Geometry: final body of the model. Coordinates: model frame, mm. Face numbers are marked on the shaded views. A direction names the side the tool comes from. Give positions to 0.01 mm unless a question says otherwise; leave off trailing zeros. Order: outer loops, then holes, each group sorted by start corner. A loop starts at its lowest first (then second) coordinate and runs counter-clockwise, first axis right, second up. Notation, with made-up numbers: (28.5, 45) -> (52.5, 45) arc R6 cw to (52.5, 50) -> close; hole circle Ø1 at (-7, 35.25). An arc over 180 degrees is marked (long way). One line per item, written item: value. Start each with the question number.
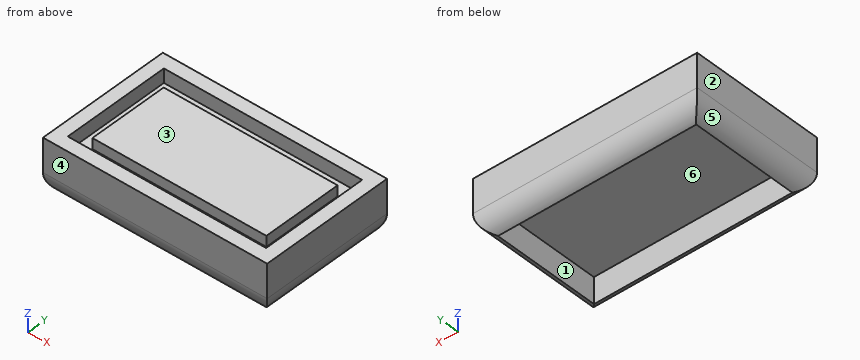
```python
from build123d import *

# Parameters (mm, degrees)
F0_W        = 50.8
F0_H        = 30.48
F0_W_2      = 44.9317246675
F0_H_2      = 24.4365520775
F1_DEPTH    = 6.35
F0_W_3      = 39.4137948751
F0_H_3      = 18.13034527
F2_DEPTH    = 3.175
F3_DEPTH    = 5.588
F4_T1_DEPTH = 76.2
F4_T3_DEPTH = 55.88


# Not quite as in the source:
# - a fillet or chamfer that OpenCascade refuses, or shapes differently, is made with other operations: its cross-section is extruded or revolved along the edge and cut away or added


with BuildPart() as f1:
    # F0 (on Top) → F1 (new body, symmetric)
    with BuildSketch(Plane.XY):
        Rectangle(F0_W, F0_H)
        Rectangle(F0_W_2, F0_H_2, mode=Mode.SUBTRACT)
    extrude(amount=F1_DEPTH, both=True)

    # F0 (on Top) → F2 (join)
    with BuildSketch(Plane.XY):
        Rectangle(F0_W_2, F0_H_2)
        Rectangle(F0_W_3, F0_H_3, mode=Mode.SUBTRACT)
    extrude(amount=F2_DEPTH)

    # F0 (on Top) → F3 (join)
    with BuildSketch(Plane.XY):
        Rectangle(F0_W_3, F0_H_3)
    extrude(amount=F3_DEPTH)

    # F4: fillet of radius 5.08 on 4 edges, made by hand

    # F4_s2 → F4_t1 (cut)
    with BuildSketch(Plane.YZ.offset(-38.1)):
        with BuildLine():
            ThreePointArc((-10.16, -6.35), (-13.7521024484, -4.8621024484), (-15.24, -1.27))
            Line((-15.24, -1.27), (-15.24, -6.35))
            Line((-15.24, -6.35), (-10.16, -6.35))
        make_face()
        with BuildLine():
            ThreePointArc((10.16, -6.35), (13.7521024484, -4.8621024484), (15.24, -1.27))
            Line((15.24, -1.27), (15.24, -6.35))
            Line((15.24, -6.35), (10.16, -6.35))
        make_face()
    extrude(amount=F4_T1_DEPTH, mode=Mode.SUBTRACT)

    # F4_s4 → F4_t3 (cut)
    with BuildSketch(Plane.XZ.offset(-27.94)):
        with BuildLine():
            ThreePointArc((25.4, -1.27), (23.9121024484, -4.8621024484), (20.32, -6.35))
            Line((20.32, -6.35), (25.4, -6.35))
            Line((25.4, -6.35), (25.4, -1.27))
        make_face()
        with BuildLine():
            ThreePointArc((-20.32, -6.35), (-23.9121024484, -4.8621024484), (-25.4, -1.27))
            Line((-25.4, -1.27), (-25.4, -6.35))
            Line((-25.4, -6.35), (-20.32, -6.35))
        make_face()
    extrude(amount=F4_T3_DEPTH, mode=Mode.SUBTRACT)


solid = f1.part
```
1. Cut plane D-D, the plane z = -4.25. Return loops of the section in (x, y).
2. Pin query (flat end, axial travel): P1, Ø14.5, axis at x = 3, y = 4, coming from the +Z side; P2, Ø2, axis at x = 1, z = -3.5, coming from the -Y side; P3, Ø5, axis at x = 17, y = 2, coming from the -Z side. Return the tip coordinate at first contact, or that it passes through.
3. Cut plane B-B, the plane x = -5.5. Return loops of the section in (y, z) (3 decimals), then the cut area to 3 significant figures.
4. Material intervals for L1, parallel to X at y = -7.5, z = 3.5; L2, parallel to Y at x = -6.5, z = 5.5; L3, parallel to X at y = -12, z = -0.25, sorted ascending. Write a range as [from, to].
5. Cut plane C-C, the plane y = -7. Return loops of the section in (x, z) (3 decimals).
6. Draft query along X for the marked faces 3, 4, 5 and 6. Return one class per face: pulls with the +X half, pulls with the -X half, needs draft (parallel to the pull), parting line crosses it, or undercut.
7. Access query for the marked faces 1 and 2. Directions: +Z, -Z, +X, -X, +Y, -Y. A direction counts if a zero-diameter tool reaches every point of the face in a straight line with its end or side. Return the directions, or none.
8. Cut plane A-A, the plane z = -0.5. Return loops of the section in (x, y).
Answers follow:
1. outline: (-24.43, -14.27) -> (24.43, -14.27) -> (24.43, 14.27) -> (-24.43, 14.27) -> close; hole (-22.47, -12.22) -> (22.47, -12.22) -> (22.47, 12.22) -> (-22.47, 12.22) -> close
2. P1: stops at z = 5.59
2. P2: stops at y = -15.09
2. P3: stops at z = 0
3. outline: (-15.24, -1.27) arc R5.08 ccw to (-12.218, -5.914) -> (-12.218, 0) -> (12.218, 0) -> (12.218, -5.914) arc R5.08 ccw to (15.24, -1.27) -> (15.24, 6.35) -> (12.218, 6.35) -> (12.218, 3.175) -> (9.065, 3.175) -> (9.065, 5.588) -> (-9.065, 5.588) -> (-9.065, 3.175) -> (-12.218, 3.175) -> (-12.218, 6.35) -> (-15.24, 6.35) -> close
3. area: 188 mm²
4. L1: x = [-25.4, -22.47], [-19.71, 19.71], [22.47, 25.4]
4. L2: y = [-15.24, -12.22], [-9.07, 9.07], [12.22, 15.24]
4. L3: x = [-25.4, -22.47], [22.47, 25.4]
5. outline: (-25.4, -1.27) arc R5.08 ccw to (-22.466, -5.875) -> (-22.466, 0) -> (22.466, 0) -> (22.466, -5.875) arc R5.08 ccw to (25.4, -1.27) -> (25.4, 6.35) -> (22.466, 6.35) -> (22.466, 3.175) -> (19.707, 3.175) -> (19.707, 5.588) -> (-19.707, 5.588) -> (-19.707, 3.175) -> (-22.466, 3.175) -> (-22.466, 6.35) -> (-25.4, 6.35) -> close
6. face 3: undercut
6. face 4: needs draft
6. face 5: pulls with the -X half
6. face 6: undercut
7. face 1: -Z
7. face 2: +Z, -Z, -X, +Y, -Y
8. outline: (-25.4, -15.24) -> (25.4, -15.24) -> (25.4, 15.24) -> (-25.4, 15.24) -> close; hole (-22.47, -12.22) -> (22.47, -12.22) -> (22.47, 12.22) -> (-22.47, 12.22) -> close
